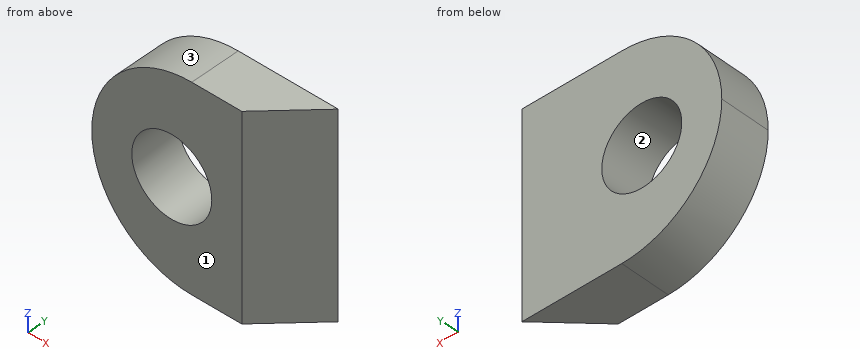
from build123d import *

# Parameters (mm, degrees)
F0_W     = 20
F0_H     = 20
F1_DEPTH = 5
F2_R     = 9.99999
F3_R     = 4
F4_DEPTH = 25
F5_SIZE  = 4.99999


# Not quite as in the source:
# - a fillet or chamfer is up to 0.001 mm smaller than in the source, because OpenCascade refuses the exact size


with BuildPart() as f1:
    # F0 (on Front) → F1 (new body)
    with BuildSketch(Plane.XZ):
        Rectangle(F0_W, F0_H)
    extrude(amount=F1_DEPTH)

    # F2 (radius 10 in the source; OpenCascade refuses exactly that, so slightly less here)
    f2_edges = [f1.edges().sort_by_distance(p)[0] for p in [
        (-10, -2.5, 10),
        (-10, -2.5, -10),
    ]]
    fillet(f2_edges, radius=F2_R)

    # F3 (on face) → F4 (cut)
    with BuildSketch(Plane.XZ.offset(5)):
        with Locations((-2, 0)):
            Circle(F3_R)
    extrude(amount=-F4_DEPTH, mode=Mode.SUBTRACT)

    # F5 (size 5 in the source; OpenCascade refuses exactly that, so slightly less here)
    f5_edges = [f1.edges().sort_by_distance(p)[0] for p in [
        (10, -5, 0),
    ]]
    chamfer(f5_edges, length=F5_SIZE)


solid = f1.part
Can you work these out from the model? Positions are in its coordinate system, mm. Face numbers are marked on the shaded views. Round coordinates to 2 decimals unless told otherwise and drop trailing zeros. Order: outer loops, then holes, each group sorted by start corner. A loop starts at its lowest first (then second) coordinate and runs counter-clockwise, first axis right, second up. Notation, with made-up numbers: (-19, 32.25) -> (24, 32.25) arc R23 cw to (24, 67.25) -> close; hole circle Ø4 at (23.5, 16). An arc over 180 degrees is marked (long way). Write each question's results on one line, items separated by ' | '. Start each with the question number.
Item 1: Thinking about a two-plate mould opening in Z: for the marked faces 1, 2 and 3, which applies, +Z half, -Z half, draft (parallel to the pull), parting line (faces both ways), or undercut?
Item 2: Please list where these lines run through material, in increasing order: L1, parallel to X at y = -3.5, z = -0.25; L2, parallel to X at y = -0.15, z = -0.5; L3, parallel to Z at x = 0.25, y = -2.55.
Item 3: If we section it at C-C, the plane x = -5.75: Write out the boundary of the cut face in (y, z), then the cut area to 3 significant figures.
Item 4: Will this pin go through, and if not, where does the flat tip stop? pin 1 (6.5 mm diameter, centred on x = -2, z = 0, fed in from +Y).
Item 5: If we section it at A-A, the plane x = -2: Write out the boundary of the cut face in (y, z), then the cut area to 3 significant figures.
Results:
1) face 1: draft | face 2: undercut | face 3: +Z half
2) L1: x = -10 to -5.99, 1.99 to 6.5 | L2: x = -9.99 to -5.97, 1.97 to 9.85 | L3: z = -10 to -3.31, 3.31 to 10
3) outline: (-5, -8.18) -> (0, -8.18) -> (0, -1.39) -> (-5, -1.39) -> close; (-5, 1.39) -> (0, 1.39) -> (0, 8.18) -> (-5, 8.18) -> close | area: 67.9 mm2
4) pin 1: passes through
5) outline: (-5, -9.8) -> (0, -9.8) -> (0, -4) -> (-5, -4) -> close; (-5, 4) -> (0, 4) -> (0, 9.8) -> (-5, 9.8) -> close | area: 58.0 mm2
